```python
from build123d import *

# Parameters (mm, degrees)
SKETCH1_W               = 88.9
SKETCH1_H               = 152.4
BOSS_EXTRUDE1_DEPTH     = 46.99
FILLET1_R               = 31.75
CUT_EXTRUDE1_DEPTH      = 143.235650654
SKETCH6_R               = 20.32
CUT_EXTRUDE2_DEPTH      = 40.64
CUT_EXTRUDE3_REACH      = 154.734
CUT_EXTRUDE3_END_RADIUS = 20.32
SKETCH14_RX             = 7.62
SKETCH14_RY             = 5.08


with BuildPart() as part:
    # Sketch1 → Boss-Extrude1 (new body)
    with BuildSketch(Plane(origin=(0, 0, 0), x_dir=(1, 0, 0), z_dir=(0, 1, 0))):
        Rectangle(SKETCH1_W, SKETCH1_H)
    extrude(amount=BOSS_EXTRUDE1_DEPTH)

    # Fillet1
    fillet1_edges = [part.edges().sort_by_distance(p)[0] for p in [
        (44.45, 23.495, 76.2),
    ]]
    fillet(fillet1_edges, radius=FILLET1_R)

    # Sketch11 → Cut-Extrude1 (cut, through all)
    with BuildSketch(Plane(origin=(18.971914377, 60.07772886, 36.046637316), x_dir=(0.9652375973044347, -0.2241263770830731, -0.13447582624984392), z_dir=(0.2613740246274715, 0.8276844113203264, 0.49661064679219535))):
        Polygon((-36.101903277, -41.164805392), (26.395662264, -50.965949533), (26.395662264, -13.939405), align=None)
    extrude(amount=CUT_EXTRUDE1_DEPTH, mode=Mode.SUBTRACT)

    # Sketch6 → Cut-Extrude2 (cut)
    with BuildSketch(Plane(origin=(0, 46.99, 0), x_dir=(1, 0, 0), z_dir=(0, 1, 0))):
        with Locations(Location((14.605, -44.45, 0), (0, 0, 270))):
            Circle(SKETCH6_R)
    extrude(amount=-CUT_EXTRUDE2_DEPTH, mode=Mode.SUBTRACT)

    # Cut-Extrude3: up to this cylinder (the profile starts outside it)
    cut_extrude3_end = Plane(origin=(14.605, 82.009764, 44.45), z_dir=(0, 1, 0)) * Cylinder(CUT_EXTRUDE3_END_RADIUS, 351.108, mode=Mode.PRIVATE)
    # Sketch14 → Cut-Extrude3 (cut, up to the surface)
    with BuildSketch(Plane(origin=(0, 65.096039324, -54.622062588), x_dir=(-1, 0, 0), z_dir=(0, 0.7660444431189772, -0.6427876096865403)), mode=Mode.PRIVATE) as cut_extrude3_sk1:
        with Locations(Location((-8.89, 26.313084008), (0, 0, 180))):
            Ellipse(SKETCH14_RX, SKETCH14_RY)
    cut_extrude3_tool1 = extrude(cut_extrude3_sk1.sketch, amount=-CUT_EXTRUDE3_REACH, mode=Mode.PRIVATE) - cut_extrude3_end
    add(cut_extrude3_tool1.solids().sort_by_distance((8.89, 82.009764, -34.465071))[0], mode=Mode.SUBTRACT)


solid = part.part
```
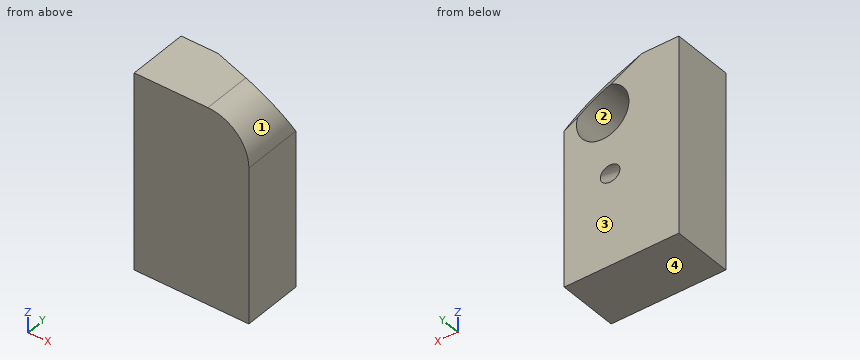
Geometry check sheet. Reference: the model listing, model coordinates, mm. Face numbers are marked on the shaded views. Give positions to 0.01 mm unless a question says otherwise; leave off trailing zeros. Order: outer loops, then holes, each group sorted by start corner. A loop starts at its lowest first (then second) coordinate and runs counter-clockwise, first axis right, second up.
1. Release check for a two-part mould opening along Z. For the marked faces 1, 2, 3 and 4 record: pulls with the +Z half, pulls with the -Z half, needs draft (parallel to the pull), parting line crosses it, or undercut.
2. Section check B-B, the plane y = 41.5. Give the number of separate pieces and of enclosed holes in the cut face, and give its area (3 significant figures).
3. Section check A-A, the plane x = 18.5. Enter the section's corners in (y, z).
4. Gauge pin test, flat ends, axial feed: pin 1 Ø1 at (x, z) = (35, -40.5) entering from -Y; pin 2 Ø2 at (x, y) = (20.5, 40.5) entering from +Z. Record the tip position at first contact, or that the pin passes through.
5. Thickness scan on L1, parallel to X at y = 31.5, z = 44.45 (3 decimals); L2, parallel to Z at x = 7, y = 32; L3, parallel to Z at x = 4.5, y = 16. Record the ranges inside material, lowest first.
Values follow:
1. face 1: pulls with the +Z half
1. face 2: undercut
1. face 3: needs draft
1. face 4: pulls with the -Z half
2. separate pieces: 1
2. enclosed holes: 2
2. area: 11,600 mm2
3. outline: (0, -76.2) - (46.99, -76.2) - (46.99, 24.51) - (6.35, 24.51) - (6.35, 64.39) - (43.22, 64.39) - (36.46, 75.67) - (0, 75.67) - close
4. pin 1: stops at y = 0
4. pin 2: stops at z = 69.62
5. L1: x = -44.45 to -5.715, 34.925 to 44.45
5. L2: z = -76.2 to 1.07, 13.92 to 25.61, 63.29 to 76.2
5. L3: z = -76.2 to 15.5, 26.34 to 26.82, 62.08 to 76.2
